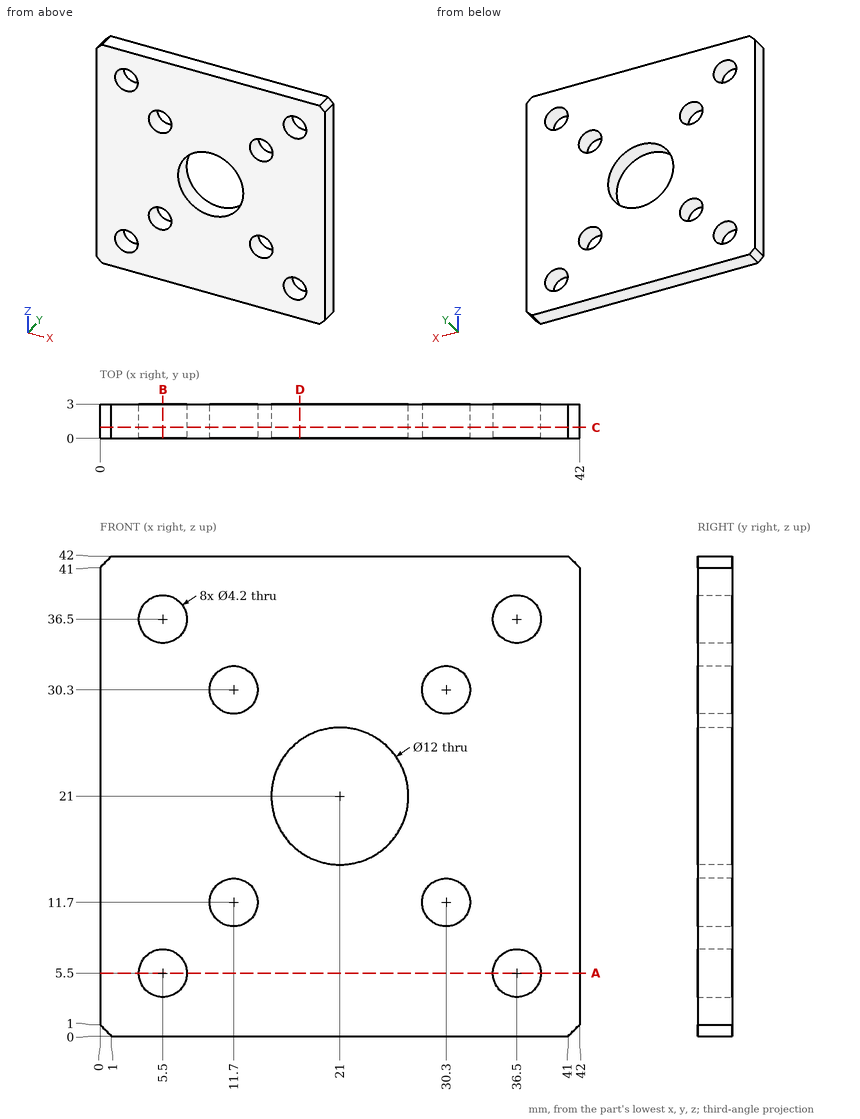
Verification items for this drawing (mm, ordinates from the low corner). Round coordinates to 2 decimals unless told otherwise and drop trailing zeros. Loops run counter-clockwise (first coordinate to the right, second up) from the corner with the lowest first, then second, coordinate; pieces in that order, holes last. Notation, with made-up numbers: (36.25, 10.25) - (85.25, 10.25) arc R15 ccw to (85.25, 16.25) - close; hole circle Ø9 at (-2, -33.75). An arc over 180 degrees is marked (long way). Write item = value, one per line.
Q1. Sectioned sample at C-C on y = 0.95. State how many separate pieces and enclosed holes the cut face has, plus the area to 3 significant figures.
Here are the results:
separate_pieces = 1
enclosed_holes = 9
area = 1,540 mm^2
Q2. Sectioned sample at B-B on x = 5.5. Record the boundary of the cut face in (y, z), plus the area to 3 significant figures.
Here are the results:
outline = (0, 0) - (3, 0) - (3, 3.4) - (0, 3.4) - close; (0, 7.6) - (3, 7.6) - (3, 34.4) - (0, 34.4) - close; (0, 38.6) - (3, 38.6) - (3, 42) - (0, 42) - close
area = 101 mm^2
Q3. Sectioned sample at A-A on z = 5.5. Record the boundary of the cut face in (x, y), plus the area to 3 significant figures.
Here are the results:
outline = (0, 0) - (3.4, 0) - (3.4, 3) - (0, 3) - close; (7.6, 0) - (34.4, 0) - (34.4, 3) - (7.6, 3) - close; (38.6, 0) - (42, 0) - (42, 3) - (38.6, 3) - close
area = 101 mm^2
Q4. Material ranges on L1, parallel to Z at x = 11.7, y = 1.7; L2, parallel to Z at x = 5.5, y = 1.65; L3, parallel to X at y = 0.45, z = 29.5, recorded low to high.
Here are the results:
L1 = 0 to 9.6, 13.8 to 28.2, 32.4 to 42
L2 = 0 to 3.4, 7.6 to 34.4, 38.6 to 42
L3 = 0 to 9.76, 13.64 to 28.36, 32.24 to 42
Q5. Sectioned sample at D-D on x = 17.5. Record the boundary of the cut face in (y, z), plus the area to 3 significant figures.
Here are the results:
outline = (0, 0) - (3, 0) - (3, 16.13) - (0, 16.13) - close; (0, 25.87) - (3, 25.87) - (3, 42) - (0, 42) - close
area = 96.8 mm^2
Q6. Depth check by flat-ended pin: pin 1 (15.5 mm diameter, centred on x = 21, z = 21, fed in from -Y). Enter the tip coordinate at first touch or a pass-through.
Here are the results:
pin_1 = 0
